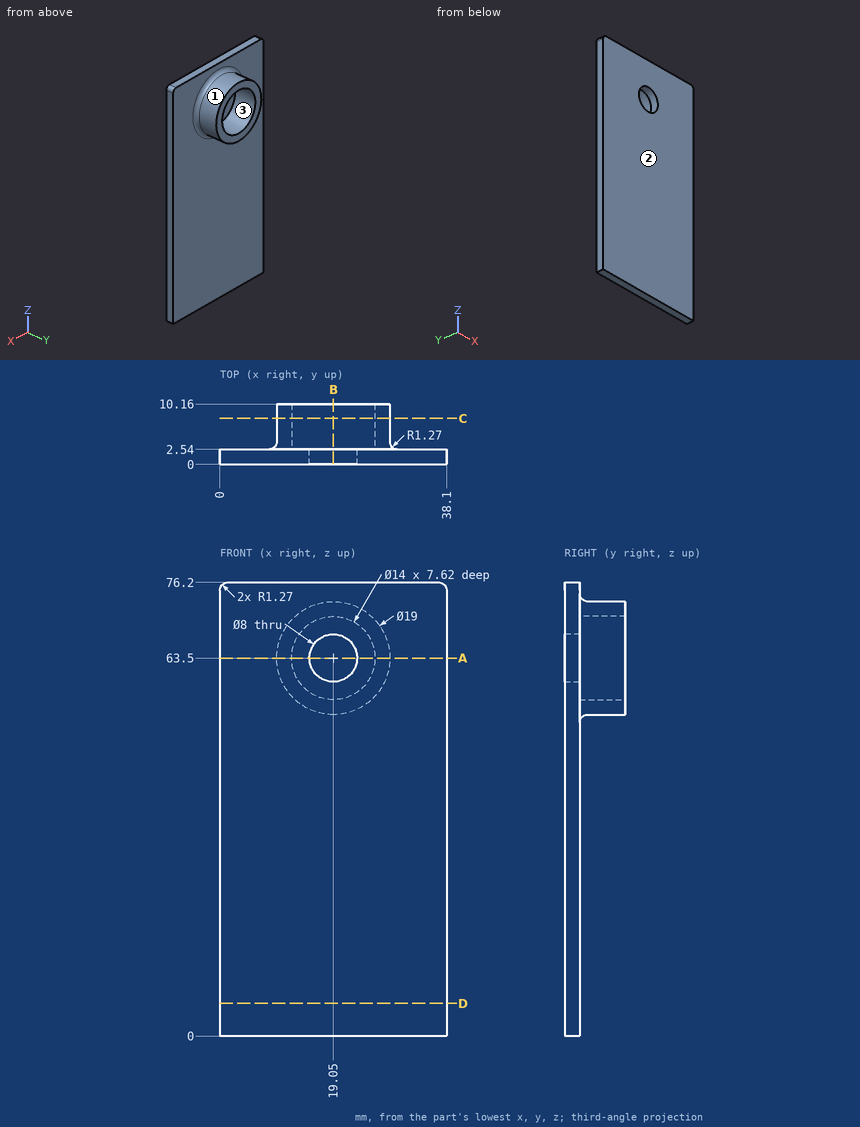
Check sheet for the drawn part. Datum: minimum x, y, z corner. Units: mm. Round coordinates to 2 decimals unless told otherwise and drop trailing zeros. Order: outer loops, then holes, each group sorted by start corner. A loop starts at its lowest first (then second) coordinate and runs counter-clockwise, first axis right, second up.
(1) Draft check along Z on the marked faces 1, 2 and 3. Enter one of: pulls with the +Z half, pulls with the -Z half, needs draft (parallel to the pull), parting line crosses it, or undercut.
(2) Go/stop test with flat-tipped pins: P1, Ø4, axis at x = 29, y = 6, coming from the -Z side; P2, Ø6, axis at x = 11.5, y = 7, coming from the +Z side. Record where each tip stops, or that it passes through.
(3) Cross-section at A-A, the plane z = 63.5. Enter the section's corners in (x, y), and give its area (3 significant figures).
(4) Scan lines: probe 1 along X at (y, z) = (2, 63.5); probe 2 along X at (y, z) = (5.5, 63.5); probe 3 along Y at (x, z) = (2.5, 73.5). Record each from-to range of solid material in increasing order.
(5) Cross-section at B-B, the plane x = 19.05. Enter the section's corners in (y, z), and give its area (3 significant figures).
(6) Cross-section at D-D, the plane z = 5.5. Enter the section's corners in (x, y), and give its area (3 significant figures).
(7) Cross-section at C-C, the plane y = 7.75. Enter the section's corners in (x, z).
Check sheet entries:
1. face 1: parting line crosses it
1. face 2: needs draft
1. face 3: undercut
2. P1: stops at z = 58.3
2. P2: stops at z = 71.84
3. outline: (0, 0) - (15.05, 0) - (15.05, 2.54) - (12.05, 2.54) - (12.05, 10.16) - (9.55, 10.16) - (9.55, 3.81) arc R1.27 cw to (8.28, 2.54) - (0, 2.54) - close; (23.05, 0) - (38.1, 0) - (38.1, 2.54) - (29.82, 2.54) arc R1.27 cw to (28.55, 3.81) - (28.55, 10.16) - (26.05, 10.16) - (26.05, 2.54) - (23.05, 2.54) - close
3. area: 115 mm2
4. probe 1: x = 0 to 15.05, 23.05 to 38.1
4. probe 2: x = 9.55 to 12.05, 26.05 to 28.55
4. probe 3: y = 0 to 2.54
5. outline: (0, 0) - (2.54, 0) - (2.54, 52.73) arc R1.27 cw to (3.81, 54) - (10.16, 54) - (10.16, 56.5) - (2.54, 56.5) - (2.54, 59.5) - (0, 59.5) - close; (0, 67.5) - (2.54, 67.5) - (2.54, 70.5) - (10.16, 70.5) - (10.16, 73) - (3.81, 73) arc R1.27 cw to (2.54, 74.27) - (2.54, 76.2) - (0, 76.2) - close
5. area: 212 mm2
6. outline: (0, 0) - (38.1, 0) - (38.1, 2.54) - (0, 2.54) - close
6. area: 96.8 mm2
7. outline: circle Ø19 at (19.05, 63.5); hole circle Ø14 at (19.05, 63.5)
